```python
from build123d import *

# Parameters (mm, degrees)
SKETCH1_W           = 220
SKETCH1_H           = 145
SKETCH1_W_2         = 42.5
SKETCH1_H_2         = 52.5
BOSS_EXTRUDE1_DEPTH = 3
SKETCH2_W           = 220
SKETCH2_H           = 145
BOSS_EXTRUDE2_DEPTH = 37
SKETCH3_W           = 27.3375
SKETCH3_H           = 19.05
CUT_EXTRUDE1_DEPTH  = 3
SKETCH3_6_W         = 53.975
SKETCH3_6_H         = 31.75
CUT_EXTRUDE2_DEPTH  = 8.5


with BuildPart() as part:
    # Sketch1 → Boss-Extrude1 (new body)
    with BuildSketch(Plane(origin=(0, 0, 0), x_dir=(1, 0, 0), z_dir=(0, 1, 0))):
        with Locations((110, 72.5)):
            Rectangle(SKETCH1_W, SKETCH1_H)
        Polygon((10, 82.5), (52.5, 82.5), (52.5, 135), (31.25, 135), (10, 108.75), align=None, mode=Mode.SUBTRACT)
        with Locations((83.75, 108.75)):
            Rectangle(SKETCH1_W_2, SKETCH1_H_2, mode=Mode.SUBTRACT)
        with Locations((83.75, 36.25)):
            Rectangle(SKETCH1_W_2, SKETCH1_H_2, mode=Mode.SUBTRACT)
        Polygon((10, 36.25), (31.25, 10), (52.5, 10), (52.5, 62.5), (10, 62.5), align=None, mode=Mode.SUBTRACT)
        Polygon((210, 62.5), (210, 36.25), (188.75, 10), (167.5, 10), (167.5, 62.5), align=None, mode=Mode.SUBTRACT)
        with Locations((136.25, 36.25)):
            Rectangle(SKETCH1_W_2, SKETCH1_H_2, mode=Mode.SUBTRACT)
        with Locations((136.25, 108.75)):
            Rectangle(SKETCH1_W_2, SKETCH1_H_2, mode=Mode.SUBTRACT)
        Polygon((210, 108.75), (188.75, 135), (167.5, 135), (167.5, 82.5), (210, 82.5), align=None, mode=Mode.SUBTRACT)
    extrude(amount=BOSS_EXTRUDE1_DEPTH)

    # Sketch2 → Boss-Extrude2 (add)
    with BuildSketch(Plane(origin=(0, 3, 0), x_dir=(1, 0, 0), z_dir=(0, 1, 0))):
        with Locations((110, 72.5)):
            Rectangle(SKETCH2_W, SKETCH2_H)
        with BuildLine():
            Line((3, 123.3), (3, 21.7))
            ThreePointArc((3, 21.7), (9.01040764, 19.21040764), (11.5, 13.2))
            Line((11.5, 13.2), (11.5, 3))
            Line((11.5, 3), (208.5, 3))
            Line((208.5, 3), (208.5, 13.2))
            ThreePointArc((208.5, 13.2), (210.98959236, 19.21040764), (217, 21.7))
            Line((217, 21.7), (217, 123.3))
            ThreePointArc((217, 123.3), (210.98959236, 125.78959236), (208.5, 131.8))
            Line((208.5, 131.8), (208.5, 142))
            Line((208.5, 142), (11.5, 142))
            Line((11.5, 142), (11.5, 131.8))
            ThreePointArc((11.5, 131.8), (9.01040764, 125.78959236), (3, 123.3))
        make_face(mode=Mode.SUBTRACT)
    extrude(amount=BOSS_EXTRUDE2_DEPTH)

    # Sketch3 → Cut-Extrude1 (cut)
    with BuildSketch(Plane.ZY.offset(-3)):
        with Locations((-35.36875, 18.478125)):
            Rectangle(SKETCH3_W, SKETCH3_H)
    extrude(amount=CUT_EXTRUDE1_DEPTH, mode=Mode.SUBTRACT)

    # Sketch3<6> → Cut-Extrude2 (cut)
    with BuildSketch(Plane.ZY.offset(-3)):
        with Locations((-29.9875, 18.875)):
            Rectangle(SKETCH3_6_W, SKETCH3_6_H)
    extrude(amount=-CUT_EXTRUDE2_DEPTH, mode=Mode.SUBTRACT)


solid = part.part
```
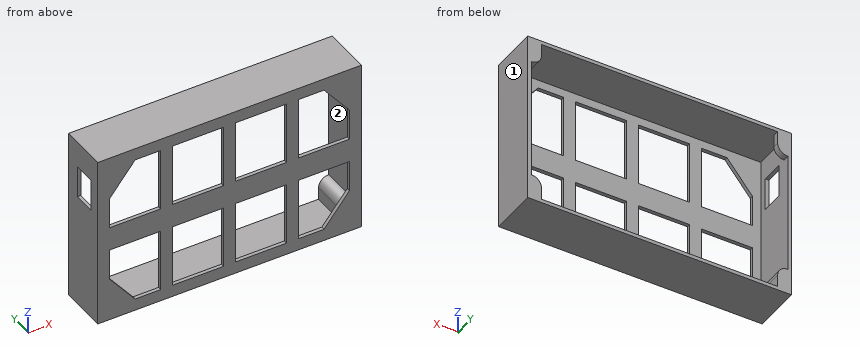
The listing builds one solid part. Answer for the finished solid, in the listing's coordinates (mm). Face numbers are marked on the shaded views. A direction names the side the tool comes from. Coordinates: 2 decimals unless noted, no trailing zeros. Loops run counter-clockwise (first coordinate to the right, second up) from the corner with the lowest first, then second, coordinate; pieces in that order, holes last. Notation, with made-up numbers: M 89.25,74 L 146.25,74 A35 ccw 146.25,110 Z; hole C 55,-22 d8. An arc over 180 degrees is marked long. Answer as CSV lines item,"result". Start each with the question number.
(1) The part is cut by section C-C (x = 146). Give the vertices of the cut face in (y, z), and give its area (3 significant figures).
(2) For the marked faces 1 and 2, determine the directions among +Z, -Z, +X, -X, +Y, -Y from which every point of the face is accessible in a straight line to the end or side of a thin tool.
(3) Find the intervals of material crossed by L1, parallel to X at y = 2, z = -43.5; L2, parallel to Z at x = 136, y = 2.5; L3, parallel to Z at x = 35, y = 11, in increasing order. Write a range as [from, to].
(4) The part is cut by section B-B (y = 13). Give the vertices of the cut face in (x, z), and give its area (3 significant figures).
(5) The part is cut by section A-A (z = -87). Give the vertices of the cut face in (x, y), and give its area (3 significant figures).
(6) The part is cut by section D-D (z = -25). Give the vertices of the cut face in (x, y), and give its area (3 significant figures).
(7) Given pin 1 (12 mm diameter, centred on x = 52.5, z = -96.5, fed in from +Y), flat-ended and moving along its own axis, determine where the tip first touches the part or whether it passes through.
Determined:
1,outline,"M 0,-145 L 40,-145 L 40,-142 L 3,-142 L 3,-135 L 0,-135 Z; M 0,-82.5 L 3,-82.5 L 3,-62.5 L 0,-62.5 Z; M 0,-10 L 3,-10 L 3,-3 L 40,-3 L 40,0 L 0,0 Z"
1,area,"342 mm2"
2,face 1,"+Z, -Z, +X, +Y, -Y"
2,face 2,"+Y"
3,L1,"[0, 10], [52.5, 62.5], [105, 115], [157.5, 167.5], [210, 220]"
3,L2,"[-145, -135], [-82.5, -62.5], [-10, 0]"
3,L3,"[-145, -142], [-3, 0]"
4,outline,"M 0,-145 L 220,-145 L 220,0 L 0,0 L 0,-21.7 L 3,-21.7 L 3,-3 L 208.5,-3 L 208.5,-13.2 A8.5 ccw 217,-21.7 L 217,-123.3 A8.5 ccw 208.5,-131.8 L 208.5,-142 L 11.5,-142 L 11.5,-131.8 A8.5 ccw 3,-123.3 L 3,-49.04 L 0,-49.04 Z"
4,area,"2,500 mm2"
5,outline,"M 0,0 L 10,0 L 10,3 L 3,3 L 3,40 L 0,40 Z; M 52.5,0 L 62.5,0 L 62.5,3 L 52.5,3 Z; M 105,0 L 115,0 L 115,3 L 105,3 Z; M 157.5,0 L 167.5,0 L 167.5,3 L 157.5,3 Z; M 210,0 L 220,0 L 220,40 L 217,40 L 217,3 L 210,3 Z"
5,area,"372 mm2"
6,outline,"M 0,0 L 19.11,0 L 19.11,3 L 3,3 L 3,8.95 L 0,8.95 Z; M 0,28 L 3,28 L 3,40 L 0,40 Z; M 52.5,0 L 62.5,0 L 62.5,3 L 52.5,3 Z; M 105,0 L 115,0 L 115,3 L 105,3 Z; M 157.5,0 L 167.5,0 L 167.5,3 L 157.5,3 Z; M 200.89,0 L 220,0 L 220,40 L 217,40 L 217,3 L 200.89,3 Z"
6,area,"369 mm2"
7,pin 1,"y = 3"
